```python
from build123d import *

# Parameters (mm, degrees)
SKETCH1_R             = 6
BOSS_EXTRUDE1_DEPTH   = 20
SKETCH2_R             = 3.175
BOSS_EXTRUDE2_DEPTH   = 25.4
SKETCH4_R             = 2.5
CUT_EXTRUDE1_DEPTH    = 6.5
F_3_0MM_DOWEL_HOLE1_D = 3


with BuildPart() as part:
    # Sketch1 → Boss-Extrude1 (new body)
    with BuildSketch(Plane(origin=(0, 0, 0), x_dir=(1, 0, 0), z_dir=(0, 1, 0))):
        with Locations(Location((0, 0, 0), (0, 0, 270))):
            Circle(SKETCH1_R)
    extrude(amount=BOSS_EXTRUDE1_DEPTH)

    # Sketch2 → Boss-Extrude2 (add)
    with BuildSketch(Plane(origin=(0, 20, 0), x_dir=(1, 0, 0), z_dir=(0, 1, 0))):
        with Locations(Location((0, 0, 0), (0, 0, 270))):
            Circle(SKETCH2_R)
    extrude(amount=BOSS_EXTRUDE2_DEPTH)

    # Sketch4 → Cut-Extrude1 (cut)
    with BuildSketch(Plane(origin=(0, 0, 0), x_dir=(-1, 0, 0), z_dir=(0, -1, 0))):
        with Locations(Location((0, 0, 0), (0, 0, 90))):
            Circle(SKETCH4_R)
    extrude(amount=-CUT_EXTRUDE1_DEPTH, mode=Mode.SUBTRACT)

    # Ø3.0mm Dowel Hole1 (through all)
    with Locations(Plane(origin=(-3.874280367, 3.174847953, 4.581479197), x_dir=(0.763579866236, 0, 0.645713394533), z_dir=(-0.645713394533, 0, 0.763579866236))):
        with Locations((0, 0)):
            Hole(F_3_0MM_DOWEL_HOLE1_D / 2)


solid = part.part
```
The listing builds one solid part. Answer for the finished solid, in the listing's coordinates (mm). A direction names the side the tool comes from. Give positions to 0.01 mm unless a question says otherwise; leave off trailing zeros. Order: outer loops, then holes, each group sorted by start corner. A loop starts at its lowest first (then second) coordinate and runs counter-clockwise, first axis right, second up. Notation, with made-up numbers: M 25,2 L 29,2 A11 cw 29,7 Z; hole C 77,-23.5 d5. An arc over 180 degrees is marked long. Put each result on its own line as item: value. Start each with the question number.
Item 1: Flat-ended cylindrical pins translate along their axes: P1, Ø1, axis at y = 35.5, z = 0, coming from the -X side (3 decimals); P2, Ø4.5, axis at x = 0, z = 0, coming from the -Y side. Find the tip coordinate at first contact, or state that the pin passes through.
Item 2: For a pull along Z with two mould halves and no side action, classify faces 1 (the face through (0, 0, 3)), 2 (the face through (0, 6.5, 0)), 3 (the face through (-1.93, 32.52, -2.52)) as +Z half, -Z half, draft (parallel to the pull), parting line (faces both ways), or undercut.
Item 3: Find the intervals of material crossed by line 1 along X through (y, z) = (2.75, 0); line 2 along Y through (x, z) = (0.25, 1.75); line 3 along Y through (x, z) = (-5, 2), in increasing order.
Item 4: Which of the six approach directions +Z, -Z, +X, -X, +Y, -Y give full straight-line access (tool end or side, diameter ignored) to faces 4 (the face through (0, 45.4, 0)), 5 (the face through (-3, 20, 3)), 6 (the face through (0.1, 3.2, 2.5))?
Item 5: The part is cut by section C-C, the plane y = 7. Determine the outline of the cut face in (x, z), and give its area (3 significant figures).
Item 6: The part is cut by section B-B, the plane y = 23.5. Determine the outline of the cut face in (x, z) (3 decimals), and give its area (3 significant figures).
Item 7: The part is cut by section A-A, the plane z = 0. Determine the outline of the cut face in (x, y) (3 decimals), and give its area (3 significant figures).
Answer key:
1. P1: stops at x = -3.175
1. P2: stops at y = 6.5
2. face 1: draft
2. face 2: undercut
2. face 3: parting line
3. line 1: x = -6 to -2.5, 2.5 to 6
3. line 2: y = 6.5 to 45.4
3. line 3: y = 0 to 20
4. face 4: +Z, -Z, +X, -X, +Y
4. face 5: +Y
4. face 6: -Y
5. outline: C 0,0 d12
5. area: 113 mm²
6. outline: C 0,0 d6.35
6. area: 31.7 mm²
7. outline: M -6,0 L -2.5,0 L -2.5,6.5 L 2.5,6.5 L 2.5,0 L 6,0 L 6,20 L 3.175,20 L 3.175,45.4 L -3.175,45.4 L -3.175,20 L -6,20 Z
7. area: 369 mm²
